from build123d import *

# Parameters (mm, degrees)
F1_DEPTH = 22.352
F2_R     = 11.650994652
F3_W     = 25.1348185512
F3_H     = 10.701005348
F5_DEPTH = 76.326557987


with BuildPart() as f1:
    # F0 (on Top) → F1 (new body)
    with BuildSketch(Plane.XY):
        Polygon((0, 37.4846383929), (-34.6435047686, 0), (0, -37.4846383929), (34.6435047686, 0), align=None)
    extrude(amount=F1_DEPTH)

    # F2
    f2_edges = [f1.edges().sort_by_distance(p)[0] for p in [
        (-17.321752, -18.742319, 22.352),
        (17.321752, 18.742319, 22.352),
    ]]
    fillet(f2_edges, radius=F2_R)

    # F3 (on face) → F5 (cut, through all)
    with BuildSketch(Plane(origin=(-18.6842489296, 17.2680835308, 0), x_dir=(-0.6787274402, -0.7343902654, 0), z_dir=(-0.7343902654, 0.6787274402, 0))):
        with Locations((-0.7411176725, 5.350502674)):
            Rectangle(F3_W, F3_H)
    extrude(amount=-F5_DEPTH, mode=Mode.SUBTRACT)


solid = f1.part
CAD build for the part. Positions are in the model's coordinates, mm. A direction names the side the tool comes from. Round coordinates to 2 decimals unless told otherwise and drop trailing zeros. Order: outer loops, then holes, each group sorted by start corner. A loop starts at its lowest first (then second) coordinate and runs counter-clockwise, first axis right, second up. Notation, with made-up numbers: (1.25, 33) - (15.25, 33) arc R20 ccw to (15.25, 59) - close; hole circle Ø10 at (-40, 53). An arc over 180 degrees is marked (long way). Return JSON: item names as keys, results as strings.
(1) Cut at C-C (z = 17.25). Give the cut face in (x, y), then the cut area to 3 significant figures.
Answer key:
{"outline": "(-33.27, 1.48) - (1.37, -36) - (33.27, -1.48) - (-1.37, 36) - close", "area": "2,390 mm^2"}
(2) Pin check, flat tips, straight feed: pin 1 Ø1 at (y, z) = (-2.5, 14) entering from -X; pin 2 Ø4 at (y, z) = (-14, 10.5) entering from -X; pin 3 Ø3 at (y, z) = (-6, 5.5) entering from +X. Stop position of each tip, or through.
Answer key:
{"pin 1": "stops at x = -32.19", "pin 2": "stops at x = -23.55", "pin 3": "stops at x = 30.48"}
(3) Wall check: probe 1 along Z at (x, y) = (6.5, -21.5); probe 2 along Y at (x, z) = (10.5, 3). Give the ranges that are in metal, low to high. Write a range as from..to.
Answer key:
{"probe 1": "z = 10.7..22.35", "probe 2": "y = -26.12..-25.81, 8.42..26.12"}
(4) Cut at B-B (z = 13.25). Give the cut face in (x, y).
Answer key:
{"outline": "(-34.45, 0.21) - (0.19, -37.28) - (34.45, -0.21) - (-0.19, 37.28) - close"}
(5) Pull direction X, two halves, no side cores. Call faces 3 (the face through (-8.29, -8.44, 5.28)), 4 (the face through (-12, -14, 0)), 5 (the face through (-17.079, 19.005, 11.02)): +X half, -X half, draft (parallel to the pull), parting line (faces both ways), or undercut.
Answer key:
{"face 3": "undercut", "face 4": "draft", "face 5": "-X half"}
(6) Cut at A-A (z = 9.25). Give the cut face in (x, y).
Answer key:
{"outline": "(-34.64, 0) - (0, -37.48) - (10.66, -25.95) - (-26.71, 8.58) - close; (-9.65, 27.04) - (27.72, -7.49) - (34.64, 0) - (0, 37.48) - close"}
(7) Tool access for faces 1 (the face through (17.564, 18.48, 5.276)), 2 (the face through (0, 1, 10.701)): list every direction of +Z, -Z, +X, -X, +Y, -Y with a clear straight run to the whole face (end or side of a thin tool).
Answer key:
{"face 1": "+Z, -Z, +X, +Y", "face 2": "-Z"}
